```python
from build123d import *

# Parameters (mm, degrees)
SKETCH_1_R      = 2.5
EXTRUDE_1_DEPTH = 168
FILLET_1_R      = 1.5


with BuildPart() as part:
    # 草图1 → 凸台-拉伸1 (new body)
    with BuildSketch(Plane.XY):
        with BuildLine():
            Line((20, 13.6), (20, 20))
            Line((20, 20), (13.6, 20))
            Line((13.6, 20), (13.6, 19.8))
            Line((13.6, 19.8), (13.2, 19.8))
            ThreePointArc((13.2, 19.8), (13.129289322, 19.770710678), (13.1, 19.7))
            Line((13.1, 19.7), (13.1, 18.3))
            ThreePointArc((13.1, 18.3), (13.129289322, 18.229289322), (13.2, 18.2))
            Line((13.2, 18.2), (15.2, 18.2))
            ThreePointArc((15.2, 18.2), (15.412132034, 18.112132034), (15.5, 17.9))
            Line((15.5, 17.9), (15.5, 16.974873734))
            ThreePointArc((15.5, 16.974873734), (15.423879533, 16.592190302), (15.207106781, 16.267766953))
            Line((15.207106781, 16.267766953), (13.132233047, 14.192893219))
            ThreePointArc((13.132233047, 14.192893219), (12.807809698, 13.976120467), (12.425126266, 13.9))
            Line((12.425126266, 13.9), (7.574873734, 13.9))
            ThreePointArc((7.574873734, 13.9), (7.192190302, 13.976120467), (6.867766953, 14.192893219))
            Line((6.867766953, 14.192893219), (4.792893219, 16.267766953))
            ThreePointArc((4.792893219, 16.267766953), (4.576120467, 16.592190302), (4.5, 16.974873734))
            Line((4.5, 16.974873734), (4.5, 17.9))
            ThreePointArc((4.5, 17.9), (4.587867966, 18.112132034), (4.8, 18.2))
            Line((4.8, 18.2), (6.8, 18.2))
            ThreePointArc((6.8, 18.2), (6.870710678, 18.229289322), (6.9, 18.3))
            Line((6.9, 18.3), (6.9, 19.7))
            ThreePointArc((6.9, 19.7), (6.870710678, 19.770710678), (6.8, 19.8))
            Line((6.8, 19.8), (6.4, 19.8))
            Line((6.4, 19.8), (6.4, 20))
            Line((6.4, 20), (0, 20))
            Line((0, 20), (0, 13.6))
            Line((0, 13.6), (0.2, 13.6))
            Line((0.2, 13.6), (0.2, 13.2))
            ThreePointArc((0.2, 13.2), (0.229289322, 13.129289322), (0.3, 13.1))
            Line((0.3, 13.1), (1.7, 13.1))
            ThreePointArc((1.7, 13.1), (1.770710678, 13.129289322), (1.8, 13.2))
            Line((1.8, 13.2), (1.8, 15.2))
            ThreePointArc((1.8, 15.2), (1.887867966, 15.412132034), (2.1, 15.5))
            Line((2.1, 15.5), (3.025126266, 15.5))
            ThreePointArc((3.025126266, 15.5), (3.407809698, 15.423879533), (3.732233047, 15.207106781))
            Line((3.732233047, 15.207106781), (5.807106781, 13.132233047))
            ThreePointArc((5.807106781, 13.132233047), (6.023879533, 12.807809698), (6.1, 12.425126266))
            Line((6.1, 12.425126266), (6.1, 7.574873734))
            ThreePointArc((6.1, 7.574873734), (6.023879533, 7.192190302), (5.807106781, 6.867766953))
            Line((5.807106781, 6.867766953), (3.732233047, 4.792893219))
            ThreePointArc((3.732233047, 4.792893219), (3.407809698, 4.576120467), (3.025126266, 4.5))
            Line((3.025126266, 4.5), (2.1, 4.5))
            ThreePointArc((2.1, 4.5), (1.887867966, 4.587867966), (1.8, 4.8))
            Line((1.8, 4.8), (1.8, 6.8))
            ThreePointArc((1.8, 6.8), (1.770710678, 6.870710678), (1.7, 6.9))
            Line((1.7, 6.9), (0.3, 6.9))
            ThreePointArc((0.3, 6.9), (0.229289322, 6.870710678), (0.2, 6.8))
            Line((0.2, 6.8), (0.2, 6.4))
            Line((0.2, 6.4), (0, 6.4))
            Line((0, 6.4), (0, 0))
            Line((0, 0), (6.4, 0))
            Line((6.4, 0), (6.4, 0.2))
            Line((6.4, 0.2), (6.8, 0.2))
            ThreePointArc((6.8, 0.2), (6.870710678, 0.229289322), (6.9, 0.3))
            Line((6.9, 0.3), (6.9, 1.7))
            ThreePointArc((6.9, 1.7), (6.870710678, 1.770710678), (6.8, 1.8))
            Line((6.8, 1.8), (4.8, 1.8))
            ThreePointArc((4.8, 1.8), (4.587867966, 1.887867966), (4.5, 2.1))
            Line((4.5, 2.1), (4.5, 3.025126266))
            ThreePointArc((4.5, 3.025126266), (4.576120467, 3.407809698), (4.792893219, 3.732233047))
            Line((4.792893219, 3.732233047), (6.867766953, 5.807106781))
            ThreePointArc((6.867766953, 5.807106781), (7.192190302, 6.023879533), (7.574873734, 6.1))
            Line((7.574873734, 6.1), (12.425126266, 6.1))
            ThreePointArc((12.425126266, 6.1), (12.807809698, 6.023879533), (13.132233047, 5.807106781))
            Line((13.132233047, 5.807106781), (15.207106781, 3.732233047))
            ThreePointArc((15.207106781, 3.732233047), (15.423879533, 3.407809698), (15.5, 3.025126266))
            Line((15.5, 3.025126266), (15.5, 2.1))
            ThreePointArc((15.5, 2.1), (15.412132034, 1.887867966), (15.2, 1.8))
            Line((15.2, 1.8), (13.2, 1.8))
            ThreePointArc((13.2, 1.8), (13.129289322, 1.770710678), (13.1, 1.7))
            Line((13.1, 1.7), (13.1, 0.3))
            ThreePointArc((13.1, 0.3), (13.129289322, 0.229289322), (13.2, 0.2))
            Line((13.2, 0.2), (13.6, 0.2))
            Line((13.6, 0.2), (13.6, 0))
            Line((13.6, 0), (20, 0))
            Line((20, 0), (20, 6.4))
            Line((20, 6.4), (19.8, 6.4))
            Line((19.8, 6.4), (19.8, 6.8))
            ThreePointArc((19.8, 6.8), (19.770710678, 6.870710678), (19.7, 6.9))
            Line((19.7, 6.9), (18.3, 6.9))
            ThreePointArc((18.3, 6.9), (18.229289322, 6.870710678), (18.2, 6.8))
            Line((18.2, 6.8), (18.2, 4.8))
            ThreePointArc((18.2, 4.8), (18.112132034, 4.587867966), (17.9, 4.5))
            Line((17.9, 4.5), (16.974873734, 4.5))
            ThreePointArc((16.974873734, 4.5), (16.592190302, 4.576120467), (16.267766953, 4.792893219))
            Line((16.267766953, 4.792893219), (14.192893219, 6.867766953))
            ThreePointArc((14.192893219, 6.867766953), (13.976120467, 7.192190302), (13.9, 7.574873734))
            Line((13.9, 7.574873734), (13.9, 12.425126266))
            ThreePointArc((13.9, 12.425126266), (13.976120467, 12.807809698), (14.192893219, 13.132233047))
            Line((14.192893219, 13.132233047), (16.267766953, 15.207106781))
            ThreePointArc((16.267766953, 15.207106781), (16.592190302, 15.423879533), (16.974873734, 15.5))
            Line((16.974873734, 15.5), (17.9, 15.5))
            ThreePointArc((17.9, 15.5), (18.112132034, 15.412132034), (18.2, 15.2))
            Line((18.2, 15.2), (18.2, 13.2))
            ThreePointArc((18.2, 13.2), (18.229289322, 13.129289322), (18.3, 13.1))
            Line((18.3, 13.1), (19.7, 13.1))
            ThreePointArc((19.7, 13.1), (19.770710678, 13.129289322), (19.8, 13.2))
            Line((19.8, 13.2), (19.8, 13.6))
            Line((19.8, 13.6), (20, 13.6))
        make_face()
        with Locations(Location((10, 10, 0), (0, 0, 180))):
            Circle(SKETCH_1_R, mode=Mode.SUBTRACT)
    extrude(amount=EXTRUDE_1_DEPTH)

    # 圆角1
    fillet_1_edges = [part.edges().sort_by_distance(p)[0] for p in [
        (0, 0, 84),
        (0, 20, 84),
        (20, 20, 84),
        (20, 0, 84),
    ]]
    fillet(fillet_1_edges, radius=FILLET_1_R)


solid = part.part
```
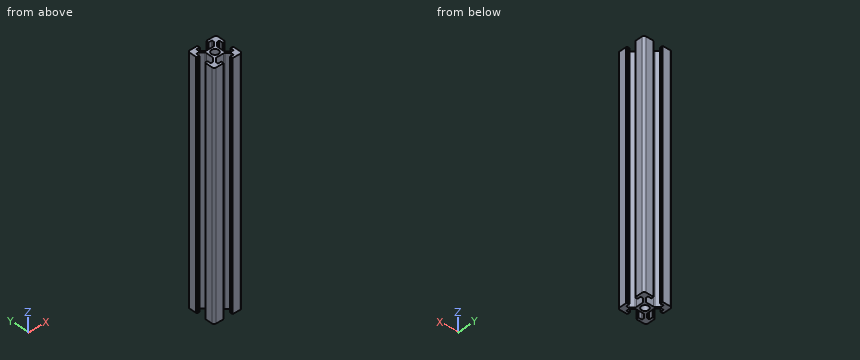
Build history of the part. All positions in model axes, mm. Coordinates: 2 decimals unless noted, no trailing zeros. Order: outer loops, then holes, each group sorted by start corner. A loop starts at its lowest first (then second) coordinate and runs counter-clockwise, first axis right, second up.
Item 1: Drill centre lines: L1, parallel to X at y = 17, z = 76; L2, parallel to X at y = 10, z = 107.5; L3, parallel to Y at x = 10.25, z = 84. Where is each one in solid material? Low to high.
Filled in:
L1: x = 0 to 4.5, 15.5 to 20
L2: x = 6.1 to 7.5, 12.5 to 13.9
L3: y = 6.1 to 7.51, 12.49 to 13.9
Item 2: Drop flat-ended pins along their axis: pin 1 Ø4 at (y, z) = (8.5, 54) entering from -X; pin 2 Ø12 at (x, y) = (10, 7) entering from -Z; pin 3 Ø0.7 at (x, z) = (0.5, 55.5) entering from -Y. Give the stop position or say it passes through.
Filled in:
pin 1: stops at x = 0.2
pin 2: stops at z = 0
pin 3: stops at y = 0.15
Item 3: Saw through at A-A on y = 10. List the corners of the cut face in (x, z).
Filled in:
outline: (6.1, 0) - (7.5, 0) - (7.5, 168) - (6.1, 168) - close; (12.5, 0) - (13.9, 0) - (13.9, 168) - (12.5, 168) - close
